```python
from build123d import *

# Parameters (mm, degrees)
SKETCH1_W           = 609.6
SKETCH1_H           = 609.6
SKETCH1_W_2         = 300
SKETCH1_H_2         = 449.2
BOSS_EXTRUDE1_DEPTH = 1.5875


with BuildPart() as part:
    # Sketch1 → Boss-Extrude1 (new body, symmetric)
    with BuildSketch(Plane(origin=(0, 0, 0), x_dir=(1, 0, 0), z_dir=(0, 1, 0))):
        Rectangle(SKETCH1_W, SKETCH1_H)
        with Locations((0, -29.4)):
            Rectangle(SKETCH1_W_2, SKETCH1_H_2, mode=Mode.SUBTRACT)
    extrude(amount=BOSS_EXTRUDE1_DEPTH, both=True)


solid = part.part
```
The model under review builds one solid part; all positions refer to its coordinate system, in mm. Round coordinates to 2 decimals unless told otherwise and drop trailing zeros. Loops run counter-clockwise (first coordinate to the right, second up) from the corner with the lowest first, then second, coordinate; pieces in that order, holes last. Notation, with made-up numbers: M -25,5 L 1,5 A19 ccw 1,28 Z; hole C 56,50 d5. An arc over 180 degrees is marked long. Put each result on its own line as item: value.
Q1. Consider section A-A, the plane x = -80. Give the boundary of the cut face in (y, z), then the cut area to 3 significant figures.
Result set:
outline: M -1.59,-304.8 L 1.59,-304.8 L 1.59,-195.2 L -1.59,-195.2 Z; M -1.59,254 L 1.59,254 L 1.59,304.8 L -1.59,304.8 Z
area: 509 mm²
Q2. Consider section C-C, the plane y = -0.1. Give the boundary of the cut face in (x, z).
Result set:
outline: M -304.8,-304.8 L 304.8,-304.8 L 304.8,304.8 L -304.8,304.8 Z; hole M -150,-195.2 L 150,-195.2 L 150,254 L -150,254 Z
Q3. Consider section B-B, the plane z = 73.5. Give the boundary of the cut face in (x, y), then the cut area to 3 significant figures.
Result set:
outline: M -304.8,-1.59 L -150,-1.59 L -150,1.59 L -304.8,1.59 Z; M 150,-1.59 L 304.8,-1.59 L 304.8,1.59 L 150,1.59 Z
area: 983 mm²
Q4. To check wall thickness, follow L1, parallel to X at y = 0.55, z = 30; L2, parallel to Z at x = -147.5, y = -0.8. State the ranges of each line that lie inside material, in increasing order.
Result set:
L1: x = -304.8 to -150, 150 to 304.8
L2: z = -304.8 to -195.2, 254 to 304.8
